Job drawing, mm, ordinate dimensions from the low corner. One solid piece. A direction names the side the tool comes from. Round coordinates to 2 decimals unless told otherwise and drop trailing zeros. Loops run counter-clockwise (first coordinate to the right, second up) from the corner with the lowest first, then second, coordinate; pieces in that order, holes last.
1) 3-axis set-ups, long thin cutter, end or side, ignore diameter. For the marked faces 4, 5 and 6: which of +Z, -Z, +X, -X, +Y, -Y reach the whole face in a straight line?
2) Drop flat-ended pins along their axis: P1, Ø0.8, axis at x = 104.5, y = 15.5, coming from the -Z side; P2, Ø5, axis at x = 119.5, y = 4.5, coming from the +Z side; P3, Ø5, axis at y = 9, z = 12.5, coming from the +X side; P4, Ø1.5, axis at x = 43, z = 3.5, coming from the -Y side. Give the stop position or say it passes through.
3) Band-saw the part on B-B, the plane y = 6. Write the cut outline in (x, z), then the cut area to 3 significant figures.
4) Mould opens along Z. For the marked faces 1, 2 and 3 say: +Z half, -Z half, draft (parallel to the pull), parting line (faces both ways), or undercut.
5) Probe line 1 (X direction, y = 14.5, z = 12); line 2 (Z direction, x = 89, y = 10.5); line 3 (Y direction, x = 29.5, z = 3.25). List the from-to ranges inside material, lowest first.
6) Band-saw the part on D-D, the plane z = 1.5. Write the cut outline in (x, y).
7) Band-saw the part on C-C, the plane x = 23. Write the cut outline in (y, z).
8) Band-saw the part on A-A, the plane z = 12.75. Write the cut outline in (x, y).
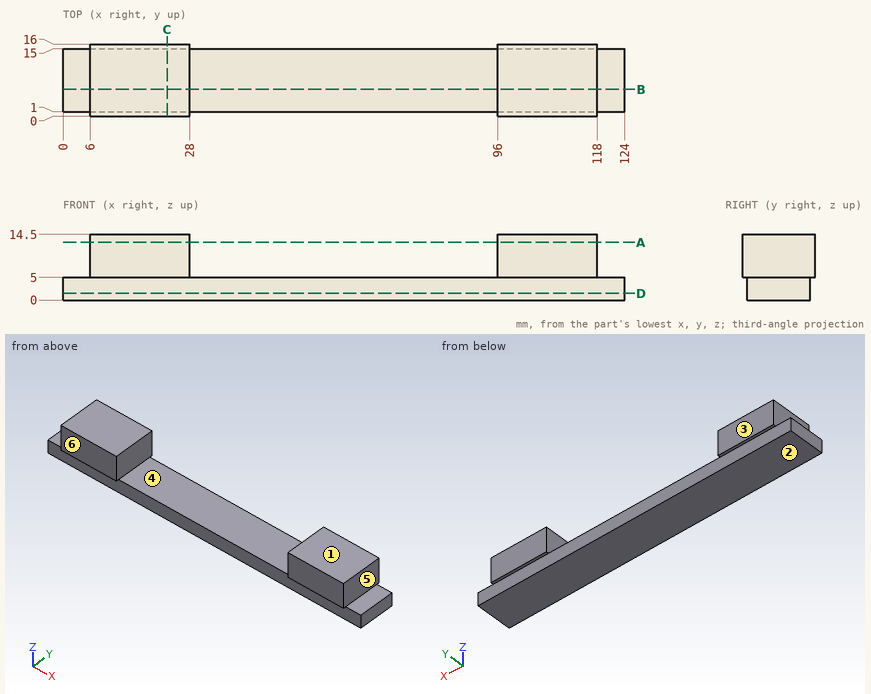
Reported:
1. face 4: +Z, +Y, -Y
1. face 5: +Z, +X, +Y, -Y
1. face 6: +Z, -Z, +X, -X, -Y
2. P1: stops at z = 5
2. P2: stops at z = 14.5
2. P3: stops at x = 118
2. P4: stops at y = 1
3. outline: (0, 0) - (124, 0) - (124, 5) - (118, 5) - (118, 14.5) - (96, 14.5) - (96, 5) - (28, 5) - (28, 14.5) - (6, 14.5) - (6, 5) - (0, 5) - close
3. area: 1,040 mm2
4. face 1: +Z half
4. face 2: -Z half
4. face 3: draft
5. line 1: x = 6 to 28, 96 to 118
5. line 2: z = 0 to 5
5. line 3: y = 1 to 15
6. outline: (0, 1) - (124, 1) - (124, 15) - (0, 15) - close
7. outline: (0, 5) - (1, 5) - (1, 0) - (15, 0) - (15, 5) - (16, 5) - (16, 14.5) - (0, 14.5) - close
8. outline: (6, 0) - (28, 0) - (28, 16) - (6, 16) - close; (96, 0) - (118, 0) - (118, 16) - (96, 16) - close
